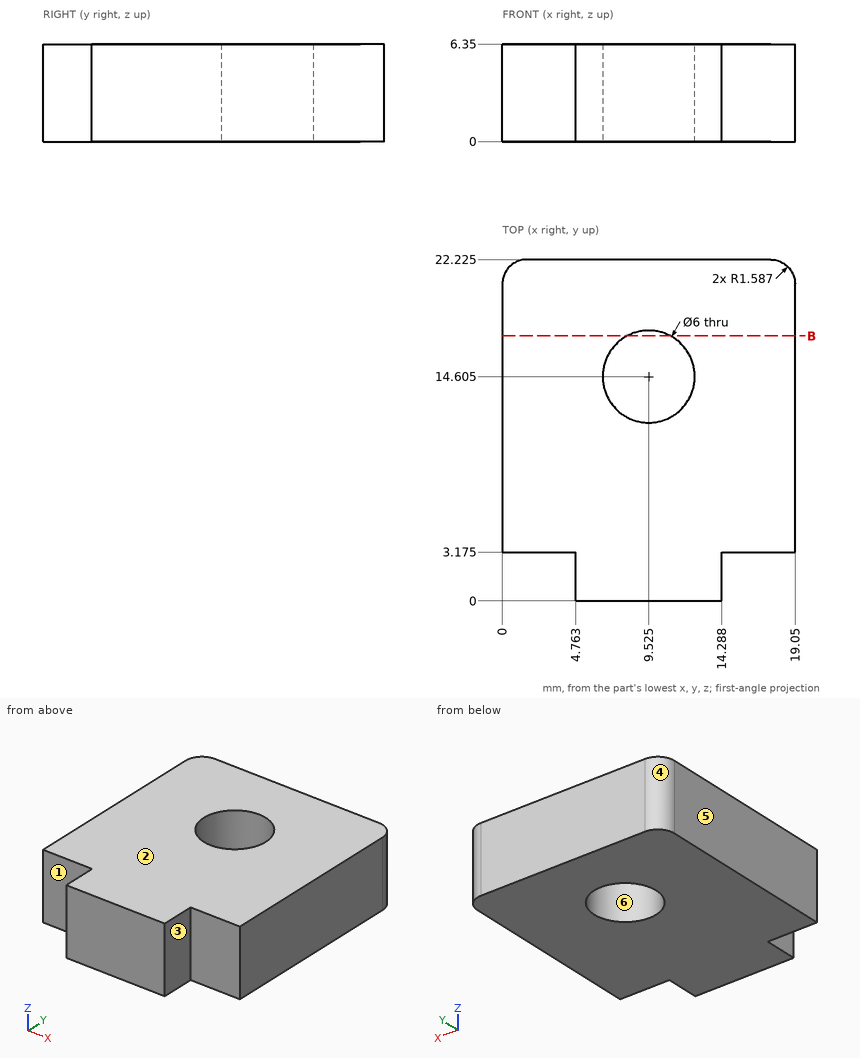
Can you work these out from the drawing? Everything is in mm from the part's minimum corner. A direction names the side the tool comes from. Give positions to 0.01 mm unless a question says otherwise; leave off trailing zeros. Write each loop counter-clockwise with the first axis right and the second up, starting at its lowest first coordinate (ties: lowest second). Pieces come first, ordered by that corner, then holes. Notation, with made-up numbers: M 33.25,49 L 43.25,49 A13 cw 43.25,58 Z; hole C 26.5,48 d1. An arc over 180 degrees is marked long. Answer in a Markdown table with one row per item. Add a question column.
Item 1: On a 3-axis mill with a long thin cutter (end or side, diameter ignored), from which of +Z, -Z, +X, -X, +Y, -Y can I reach the whole of each face in a straight line? I mean the marked faces 1, 2 and 3. Say none if no direction works.
Item 2: We'd pull the mould along Y, two halves only. Please class the marked faces 4, 5 and 6: released by +Y, released by -Y, zero draft, split by the parting line, or undercut.
Item 3: Imagine slicing it at B-B, the plane y = 17.25. Write out the boundary of the cut face in (x, z).
Item 4: Please list where these lines run through material, in increasing order: L1, parallel to X at y = 14.5, z = 3.25; L2, parallel to Y at x = 1.5, z = 5.75 (1 decimal); L3, parallel to Y at x = 10.5, z = 5.5 (1 decimal).
Item 5: For pin 1 Ø1 at (y, z) = (2, 4) entering from +X; pin 2 Ø1.4 at (x, z) = (16, 3.5) entering from -Y (1 decimal), each with a flat end and sliding along its axis, tell me the tip position at first contact or that it passes through.
Evaluation:
| question | item | result |
|---|---|---|
| 1 | face 1 | +Z, -Z, -X, -Y |
| 1 | face 2 | +Z, +X, -X, +Y, -Y |
| 1 | face 3 | +Z, -Z, +X, -Y |
| 2 | face 4 | released by +Y |
| 2 | face 5 | zero draft |
| 2 | face 6 | undercut |
| 3 | outline | M 0,0 L 8.11,0 L 8.11,6.35 L 0,6.35 Z; M 10.94,0 L 19.05,0 L 19.05,6.35 L 10.94,6.35 Z |
| 4 | L1 | x = 0 to 6.53, 12.52 to 19.05 |
| 4 | L2 | y = 3.2 to 22.2 |
| 4 | L3 | y = 0 to 11.8, 17.4 to 22.2 |
| 5 | pin 1 | stops at x = 14.29 |
| 5 | pin 2 | stops at y = 3.2 |
